Can you work these out from the model? Positions are in its coordinate system, mm. A direction names the side the tool comes from. Round coordinates to 2 decimals unless told otherwise and drop trailing zeros. Order: outer loops, then holes, each group sorted by start corner. A loop starts at its lowest first (then second) coordinate and runs counter-clockwise, first axis right, second up. Notation, with made-up numbers: (12, -40) -> (30, -40) arc R8 cw to (30, -34) -> close; hole circle Ø6 at (84, 11). An arc over 180 degrees is marked (long way). Use a Markdown table: item, result. Add a question column.
Q1. If we section it at A-A on x = 1.25: List the corners of the cut face in (y, z) for me, plus the area to 3 significant figures.
Q2. I need wall thicknesses on line 1 along Y through (x, z) = (-16, 16); line 2 along Z through (x, y) = (-15.5, -15); line 3 along X through (y, z) = (0.5, 7). Which ranges of each line are inside material? Lowest first, please. Write a range as [from, to].
Q3. If we section it at C-C on y = 7: List the corners of the cut face in (x, z) for me.
Q4. If we section it at B-B on x = -17.5: List the corners of the cut face in (y, z) for me, plus the area to 3 significant figures.
Q5. We'd pull the mould along Y, two halves only. Please class faces 4 (the face through (-8, -22.5, 5)), 5 (the face through (-14.93, -16.743, -14.889)), 6 (the face through (-20, 0, 0)), 7 (the face through (-9, 15, -16.4)): +Y half, -Y half, draft (parallel to the pull), parting line (faces both ways), or undercut.
Q6. For faces 1 (the face through (8.808, -0.315, 3.262)), 2 (the face through (-14.93, 13.257, -14.889)), 3 (the face through (-5, 0, 22.5)), which set-ups out of +Z, -Z, +X, -X, +Y, -Y let a thin tool reach every point of the face, with its end or its side?
Q7. If we section it at D-D on z = 5.5: List the corners of the cut face in (x, y) for me, plus the area to 3 significant figures.
Q8. I'm going to push flat-ended pins straight in: pin 1 Ø1 at (x, z) = (-6.5, 2) entering from +Y; pin 2 Ø2.5 at (y, z) = (15, 16) entering from -X; pin 3 Ø3.5 at (y, z) = (-15, 16) entering from -X. Where does each tip first touch, or does it pass through?
Autodesk Inventor part; units mm, degrees
ref_plane "YZ Plane" through (0, 0, 0) normal (1, 0, 0) x (0, 1, 0)
ref_plane "XZ Plane" through (0, 0, 0) normal (0, 1, 0) x (-1, 0, 0)
ref_plane "XY Plane" through (0, 0, 0) normal (0, 0, 1) x (1, 0, 0)
sketch "スケッチ1" plane through (0, 0, 0) normal (0, 1, 0) x (-1, 0, 0)
  arc A0 (-7.5813, -2.554) -> (-7.5813, 2.554) centre (0, 0) ccw
  line L0 (-10, -3.9505) -> (-7.5813, -2.554)
  line L1 (20, 0) -> (20, -22.5)
  line L2 (20, -22.5) -> (-10, -22.5)
  line L3 (-10, -22.5) -> (-10, -3.9505)
  line L4 (-10, 3.9505) -> (-7.5813, 2.554)
  line L5 (20, 0) -> (20, 22.5)
  line L6 (20, 22.5) -> (-10, 22.5)
  line L7 (-10, 22.5) -> (-10, 3.9505)
  dimension "d4" = 16
  dimension "d8" = 20
  dimension "d9" = 22.5
  dimension "d10" = 30
extrude "押し出し1" add sketch "スケッチ1" along normal mid plane 45
sketch "スケッチ2" plane through (-20, -22.5, -22.5) normal (-1, 0, 0) x (0, 0, 1)
  line L0 (45, 0) -> (45, 45)
  line L1 (0, 45) -> (45, 45)
  line L2 (45, 0) -> (0, 0)
  line L3 (22.5, 22.5) -> (22.5, 37.5)
  line L4 (22.5, 37.5) -> (38.5, 37.5)
  line L5 (22.5, 22.5) -> (0, 22.5)
  point P0 (6.5, 37.5)
  point P1 (38.5, 7.5)
  point P2 (6.5, 7.5)
  dimension "d13" = 15
  dimension "d14" = 16
hole "穴1" at (-20, 15, 16) at (-20, 15, -16) at (-20, -15, 16) at (-20, -15, -16) direction (1, 0, 0) diameter 4.134 depth 10 tip angle 118
properties part number "linearbearing" material "ステンレス鋼 440C"
Answer below:
| question | item | result |
|---|---|---|
| 1 | outline | (-22.5, -22.5) -> (22.5, -22.5) -> (22.5, -7.9) -> (-22.5, -7.9) -> close; (-22.5, 7.9) -> (22.5, 7.9) -> (22.5, 22.5) -> (-22.5, 22.5) -> close |
| 1 | area | 1,310 mm² |
| 2 | line 1 | [-22.5, -17.07], [-12.93, 12.93], [17.07, 22.5] |
| 2 | line 2 | [-22.5, -18.07], [-13.93, 13.93], [18.07, 22.5] |
| 2 | line 3 | [-20, -3.87], [3.87, 10] |
| 3 | outline | (-20, -22.5) -> (10, -22.5) -> (10, -3.95) -> (7.58, -2.55) arc R8 cw (long way) to (7.58, 2.55) -> (10, 3.95) -> (10, 22.5) -> (-20, 22.5) -> close |
| 4 | outline | (-22.5, -22.5) -> (22.5, -22.5) -> (22.5, 22.5) -> (-22.5, 22.5) -> close; hole circle Ø4.13 at (-15, -16); hole circle Ø4.13 at (-15, 16); hole circle Ø4.13 at (15, -16); hole circle Ø4.13 at (15, 16) |
| 4 | area | 1,970 mm² |
| 5 | face 4 | -Y half |
| 5 | face 5 | undercut |
| 5 | face 6 | draft |
| 5 | face 7 | undercut |
| 6 | face 1 | +X, +Y, -Y |
| 6 | face 2 | -X |
| 6 | face 3 | +Z, +X, -X, +Y, -Y |
| 7 | outline | (-20, -22.5) -> (-5.81, -22.5) -> (-5.81, 22.5) -> (-20, 22.5) -> close; (5.81, -22.5) -> (10, -22.5) -> (10, 22.5) -> (5.81, 22.5) -> close |
| 7 | area | 827 mm² |
| 8 | pin 1 | through |
| 8 | pin 2 | x = -9.51 |
| 8 | pin 3 | x = -9.81 |
